Work out the finished part from the listing and answer in its coordinate system (mm). Face numbers are marked on the shaded views. A direction names the side the tool comes from. Coordinates: 2 decimals unless noted, no trailing zeros. Loops run counter-clockwise (first coordinate to the right, second up) from the corner with the lowest first, then second, coordinate; pieces in that order, holes last.
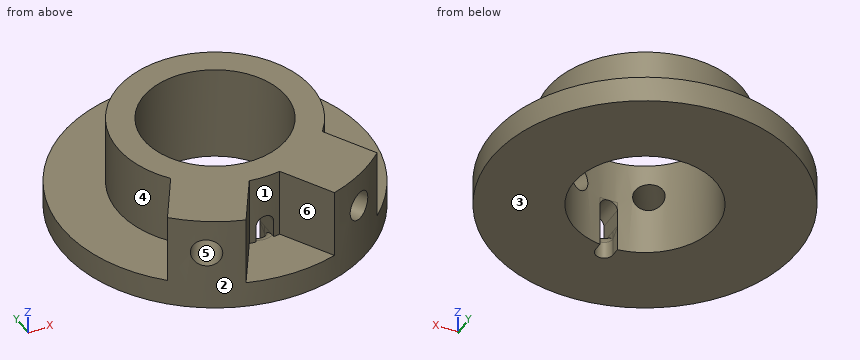
```python
from build123d import *

# Parameters (mm, degrees)
SKETCH1_R                            = 17.5
SKETCH1_R_2                          = 8.15
BOSS_EXTRUDE1_DEPTH                  = 3
SKETCH2_R                            = 11.15
SKETCH2_R_2                          = 8.15
BOSS_EXTRUDE2_DEPTH                  = 8
BOSS_EXTRUDE5_REACH                  = 39.295
BOSS_EXTRUDE5_END_RADIUS             = 17.5
SKETCH4_W                            = 8
SKETCH4_H                            = 8
BOSS_EXTRUDE5_DIRECTION_2_REACH      = 39.295
BOSS_EXTRUDE5_DIRECTION_2_END_RADIUS = 11.15
CUT_EXTRUDE1_REACH                   = 39.295
CUT_EXTRUDE1_END_RADIUS              = 8.15
SKETCH3_R                            = 1.65
CUT_EXTRUDE1_DIRECTION_2_REACH       = 39.295
CUT_EXTRUDE1_DIRECTION_2_END_RADIUS  = 17.5
CUT_EXTRUDE2_DEPTH                   = 3
CUT_EXTRUDE2_DEPTH_BACK              = 27.009613773
SKETCH6_W                            = 2
SKETCH6_H                            = 9.382987565
CUT_EXTRUDE3_DEPTH                   = 3
FILLET2_R                            = 1


with BuildPart() as part:
    # Sketch1 → Boss-Extrude1 (new body)
    with BuildSketch(Plane.XY):
        Circle(SKETCH1_R)
        Circle(SKETCH1_R_2, mode=Mode.SUBTRACT)
    extrude(amount=BOSS_EXTRUDE1_DEPTH)

    # Sketch2 → Boss-Extrude2 (add)
    with BuildSketch(Plane.XY.offset(3)):
        Circle(SKETCH2_R)
        Circle(SKETCH2_R_2, mode=Mode.SUBTRACT)
    extrude(amount=BOSS_EXTRUDE2_DEPTH)

    # Boss-Extrude5: up to this cylinder (the profile starts inside it)
    boss_extrude5_end = Plane(origin=(0, 0, 7), z_dir=(0, 0, -1)) * Cylinder(BOSS_EXTRUDE5_END_RADIUS, 114.59, mode=Mode.PRIVATE)
    # Sketch4 → Boss-Extrude5 (add, up to the surface)
    with BuildSketch(Plane(origin=(-5.575, -9.656183252, 0), x_dir=(0, 0, -1), z_dir=(-0.500000000000001, -0.866025403784438, 0)), mode=Mode.PRIVATE) as boss_extrude5_sk1:
        with Locations((-7, 0)):
            Rectangle(SKETCH4_W, SKETCH4_H)
    boss_extrude5_tool1 = extrude(boss_extrude5_sk1.sketch, amount=BOSS_EXTRUDE5_REACH, mode=Mode.PRIVATE) & boss_extrude5_end
    boss_extrude5 = boss_extrude5_tool1.solids().sort_by_distance((-5.575, -9.656183, 7))[0]
    add(boss_extrude5)

    # Boss-Extrude5 direction 2: up to this cylinder (the profile starts outside it)
    boss_extrude5_direction_2_end = Plane(origin=(0, 0, 7), z_dir=(0, 0, -1)) * Cylinder(BOSS_EXTRUDE5_DIRECTION_2_END_RADIUS, 101.89, mode=Mode.PRIVATE)
    # Sketch4 → Boss-Extrude5 direction 2 (add, up to the surface)
    with BuildSketch(Plane(origin=(-5.575, -9.656183252, 0), x_dir=(0, 0, -1), z_dir=(-0.500000000000001, -0.866025403784438, 0)), mode=Mode.PRIVATE) as boss_extrude5_direction_2_sk1:
        with Locations((-7, 0)):
            Rectangle(SKETCH4_W, SKETCH4_H)
    boss_extrude5_direction_2_tool1 = extrude(boss_extrude5_direction_2_sk1.sketch, amount=-BOSS_EXTRUDE5_DIRECTION_2_REACH, mode=Mode.PRIVATE) - boss_extrude5_direction_2_end
    boss_extrude5_direction_2 = boss_extrude5_direction_2_tool1.solids().sort_by_distance((-5.575, -9.656183, 7))[0] + boss_extrude5_direction_2_tool1.solids().sort_by_distance((-5.575, -9.656183, 7))[1]
    add(boss_extrude5_direction_2)
    boss_extrude5 = boss_extrude5 + boss_extrude5_direction_2  # both directions under the feature's name, for the pattern or mirror that repeats it

    # Cut-Extrude1: up to this cylinder (the profile starts outside it)
    cut_extrude1_end = Plane(origin=(0, 0, 7), z_dir=(0, 0, -1)) * Cylinder(CUT_EXTRUDE1_END_RADIUS, 95.89, mode=Mode.PRIVATE)
    # Sketch3 → Cut-Extrude1 (cut, up to the surface)
    with BuildSketch(Plane(origin=(-5.575, -9.656183252, 0), x_dir=(0, 0, -1), z_dir=(-0.500000000000001, -0.866025403784438, 0)), mode=Mode.PRIVATE) as cut_extrude1_sk1:
        with Locations(Location((-7, 0, 0), (0, 0, 90))):
            Circle(SKETCH3_R)
    cut_extrude1_tool1 = extrude(cut_extrude1_sk1.sketch, amount=-CUT_EXTRUDE1_REACH, mode=Mode.PRIVATE) - cut_extrude1_end
    cut_extrude1 = cut_extrude1_tool1.solids().sort_by_distance((-5.575, -9.656183, 7))[0]
    add(cut_extrude1, mode=Mode.SUBTRACT)

    # Cut-Extrude1 direction 2: up to this cylinder (the profile starts inside it)
    cut_extrude1_direction_2_end = Plane(origin=(0, 0, 7), z_dir=(0, 0, -1)) * Cylinder(CUT_EXTRUDE1_DIRECTION_2_END_RADIUS, 114.59, mode=Mode.PRIVATE)
    # Sketch3 → Cut-Extrude1 direction 2 (cut, up to the surface)
    with BuildSketch(Plane(origin=(-5.575, -9.656183252, 0), x_dir=(0, 0, -1), z_dir=(-0.500000000000001, -0.866025403784438, 0)), mode=Mode.PRIVATE) as cut_extrude1_direction_2_sk1:
        with Locations(Location((-7, 0, 0), (0, 0, 90))):
            Circle(SKETCH3_R)
    cut_extrude1_direction_2_tool1 = extrude(cut_extrude1_direction_2_sk1.sketch, amount=CUT_EXTRUDE1_DIRECTION_2_REACH, mode=Mode.PRIVATE) & cut_extrude1_direction_2_end
    cut_extrude1_direction_2 = cut_extrude1_direction_2_tool1.solids().sort_by_distance((-5.575, -9.656183, 7))[0]
    add(cut_extrude1_direction_2, mode=Mode.SUBTRACT)
    cut_extrude1 = cut_extrude1 + cut_extrude1_direction_2  # both directions under the feature's name, for the pattern or mirror that repeats it

    # Mirror1: Boss-Extrude5, Cut-Extrude1 across plane
    add(boss_extrude5.mirror(Plane(origin=(0, 0, 0), x_dir=(0, 0, 1), z_dir=(1, 0, 0))))
    add(cut_extrude1.mirror(Plane(origin=(0, 0, 0), x_dir=(0, 0, 1), z_dir=(1, 0, 0))), mode=Mode.SUBTRACT)

    # Sketch5 → Cut-Extrude2 (cut, two sides: drawn at the far end of the back side and taken through both)
    with BuildSketch(Plane.XY.offset(3).offset(-CUT_EXTRUDE2_DEPTH_BACK)):
        with BuildLine():
            Line((-1, -9.088417645), (-1, -8.088417645))
            Line((-1, -8.088417645), (1, -8.088417645))
            Line((1, -8.088417645), (1, -9.088417645))
            ThreePointArc((1, -9.088417645), (0, -10.088417645), (-1, -9.088417645))
        make_face()
    extrude(amount=CUT_EXTRUDE2_DEPTH + CUT_EXTRUDE2_DEPTH_BACK, mode=Mode.SUBTRACT)

    # Sketch6 → Cut-Extrude3 (cut)
    with BuildSketch(Plane.XY.offset(3)):
        with Locations((0, -12.779911428)):
            Rectangle(SKETCH6_W, SKETCH6_H)
    extrude(amount=CUT_EXTRUDE3_DEPTH, mode=Mode.SUBTRACT)

    # Fillet2
    # the kernel refuses this fillet: 1 mm, written as the material it adds along each edge
    with BuildSketch(Plane(origin=(1, -9.088417645, 6), x_dir=(0, 0, -1), z_dir=(0, -1, 0))) as fillet2_piece_1_section:
        with BuildLine():
            CenterArc((FILLET2_R, -FILLET2_R), FILLET2_R, 90, 90)
            Line((0, -FILLET2_R), (0, 0))
            Line((0, 0), (FILLET2_R, 0))
        make_face()
    fillet2_piece_1 = extrude(amount=4.516648766, mode=Mode.PRIVATE)
    fillet2_piece_1 = fillet2_piece_1 & Plane(origin=(0, 0, 5.777290132), x_dir=(1, 0, 0), z_dir=(0, 0, -1)) * Cylinder(11.15, 14, mode=Mode.PRIVATE)
    add(fillet2_piece_1)
    with BuildSketch(Plane(origin=(-1, -13.605066411, 6), x_dir=(1, 0, 0), z_dir=(0, 1, 0))) as fillet2_piece_2_section:
        with BuildLine():
            CenterArc((FILLET2_R, FILLET2_R), FILLET2_R, 180, 90)
            Line((0, FILLET2_R), (0, 0))
            Line((0, 0), (FILLET2_R, 0))
        make_face()
    fillet2_piece_2 = extrude(amount=4.516648766, mode=Mode.PRIVATE)
    fillet2_piece_2 = fillet2_piece_2 & Plane(origin=(0, 0, 5.777290055), x_dir=(1, 0, 0), z_dir=(0, 0, -1)) * Cylinder(11.15, 14, mode=Mode.PRIVATE)
    add(fillet2_piece_2)
    with BuildSketch(Plane(origin=(-1, -9.088417645, 6), x_dir=(1, 0, 0), z_dir=(0, 1, 0))) as fillet2_piece_3_section:
        with BuildLine():
            CenterArc((FILLET2_R, FILLET2_R), FILLET2_R, 180, 90)
            Line((0, FILLET2_R), (0, 0))
            Line((0, 0), (FILLET2_R, 0))
        make_face()
    fillet2_piece_3 = extrude(amount=3.5, mode=Mode.PRIVATE)
    fillet2_piece_3 = fillet2_piece_3 - Plane(origin=(0, 0, 5.774756303), x_dir=(1, 0, 0), z_dir=(0, 0, -1)) * Cylinder(8.15, 12, mode=Mode.PRIVATE)
    add(fillet2_piece_3)
    with BuildSketch(Plane(origin=(1, -5.588417645, 6), x_dir=(0, 0, -1), z_dir=(0, -1, 0))) as fillet2_piece_4_section:
        with BuildLine():
            CenterArc((FILLET2_R, -FILLET2_R), FILLET2_R, 90, 90)
            Line((0, -FILLET2_R), (0, 0))
            Line((0, 0), (FILLET2_R, 0))
        make_face()
    fillet2_piece_4 = extrude(amount=3.5, mode=Mode.PRIVATE)
    fillet2_piece_4 = fillet2_piece_4 - Plane(origin=(0, 0, 5.77475637), x_dir=(1, 0, 0), z_dir=(0, 0, -1)) * Cylinder(8.15, 12, mode=Mode.PRIVATE)
    add(fillet2_piece_4)
    # the kernel refuses this fillet: 1 mm, written as the material it takes off along each edge
    with BuildSketch(Plane(origin=(0, -9.088417645, 3), x_dir=(0.003141587485879873, 0.9999950652018583, 0), z_dir=(-0.9999950652018583, 0.003141587485879873, 0))) as fillet2_2_piece_1_section:
        with BuildLine():
            CenterArc((1 + FILLET2_R, FILLET2_R), FILLET2_R, 180, 90)
            Line((1 + FILLET2_R, 0), (1, 0))
            Line((1, 0), (1, FILLET2_R))
        make_face()
    fillet2_2_piece_1 = revolve(axis=Axis((0, -9.088417645, 3), (0, 0, -1)), revolution_arc=359.64, mode=Mode.PRIVATE)
    fillet2_2_piece_1 = split(fillet2_2_piece_1, bisect_by=Plane(origin=(1, -10.091717807, 2.766201228), z_dir=(-1, 0, 0)), keep=Keep.TOP, mode=Mode.PRIVATE)
    fillet2_2_piece_1 = split(fillet2_2_piece_1, bisect_by=Plane(origin=(-1, -10.091717807, 2.766201228), z_dir=(1, 0, 0)), keep=Keep.TOP, mode=Mode.PRIVATE)
    add(fillet2_2_piece_1, mode=Mode.SUBTRACT)


solid = part.part
```
1. A cutting plane is placed at B-B, the plane z = 1.5. Give the vertices of the cut face in (x, y).
2. A cutting plane is placed at A-A, the plane y = 0. Give the vertices of the cut face in (x, z).
3. Determine the mould class of the marked faces 1, 2 and 3 for opening direction X: released by +X, released by -X, zero draft, split by the parting line, or undercut.
4. Each of these flat-tipped pins is pushed along its axis until it touches: P1, Ø0.6, axis at y = -10.5, z = 3.5, coming from the +X side; P2, Ø1.5, axis at y = -12.5, z = 7, coming from the -X side; P3, Ø2, axis at y = 3.5, z = 3.5, coming from the -X side. Where does it stop, or does it pass through?
5. A cutting plane is placed at C-C, the plane x = 14. Give the vertices of the cut face in (y, z), then the cut area to 3 significant figures.
6. Straight lines are drawn through the part: probe 1 along X at (y, z) = (0, 7); probe 2 along Y at (x, z) = (-5.5, 6.25). For each, find the intervals that lie inside material, in ascending order.
7. For the marked faces 4, 5 and 6, determine the directions among +Z, -Z, +X, -X, +Y, -Y from which every point of the face is accessible in a straight line to the end or side of a thin tool.
Answers below:
1. outline: circle Ø35 at (0, 0); hole (-1, -9.09) arc R1 ccw to (1, -9.09) - (1, -8.09) arc R8.15 ccw (long way) to (-1, -8.09) - close
2. outline: (-17.5, 0) - (-8.15, 0) - (-8.15, 11) - (-11.15, 11) - (-11.15, 3) - (-17.5, 3) - close; (8.15, 0) - (17.5, 0) - (17.5, 3) - (11.15, 3) - (11.15, 11) - (8.15, 11) - close
3. face 1: undercut
3. face 2: split by the parting line
3. face 3: zero draft
4. P1: stops at x = 10.85
4. P2: stops at x = -11.98
4. P3: stops at x = -17.3
5. outline: (-10.5, 0) - (10.5, 0) - (10.5, 3) - (-10.5, 3) - close
5. area: 63.0 mm2
6. probe 1: x = -11.15 to -8.15, 8.15 to 11.15
6. probe 2: y = -16.61 to -12.47, -6.59 to -6.01, 6.01 to 9.7
7. face 4: +Z
7. face 5: none
7. face 6: +Z, -Y
